Could you check a few things on this model? Use its own coordinates, in mm. Coordinates: 2 decimals unless noted, no trailing zeros. Write each loop counter-clockwise with the first axis right and the second up, starting at its lowest first coordinate (ties: lowest second). Pieces come first, ordered by that corner, then holes. Notation, with made-up numbers: (86, -21) - (125, -21) arc R30 cw to (125, 8) - close; hole circle Ø2 at (20.25, 53). An arc over 180 degrees is marked (long way). Answer as a JSON object with one key per item and string values. Group by question number.
1) Please list where these lines run through material, in increasing order: line 1 along X through (y, z) = (1.85, 0); line 2 along Z through (x, y) = (45, 1.2); line 3 along X through (y, z) = (1.6, 1.5).
2) If we section it at B-B (y = 1.8): Write out the boundary of the cut face in (x, z).
3) Will this pin go through, and if not, where does the flat tip stop? pin 1 Ø6.5 at (x, z) = (45, 0) entering from +Y.
4) If we section it at A-A (z = 0): Write out the boundary of the cut face in (x, y), plus the area to 3 significant figures.
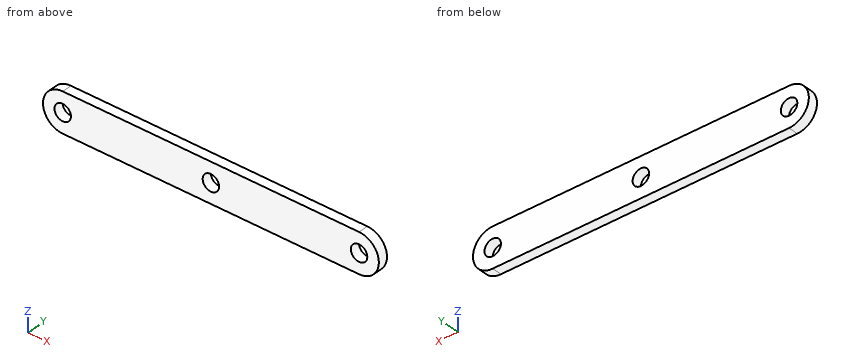
```python
from build123d import *

# Parameters (mm, degrees)
EXTRUDE_1_DEPTH     = 3
CUT_EXTRUDE_1_REACH = 5
SKETCH_2_R          = 2.5


with BuildPart() as part:
    # 草圖1 → 填料-伸長1 (new body)
    with BuildSketch(Plane(origin=(0, 0, 0), x_dir=(1, 0, 0), z_dir=(0, 1, 0))):
        with BuildLine():
            Line((-45, 6), (45, 6))
            ThreePointArc((45, 6), (51, 0), (45, -6))
            Line((45, -6), (-45, -6))
            ThreePointArc((-45, -6), (-51, 0), (-45, 6))
        make_face()
    extrude(amount=EXTRUDE_1_DEPTH)

    # 草圖2 → 除料-伸長1 (cut, up to next)
    with BuildSketch(Plane(origin=(0, 3, 0), x_dir=(1, 0, 0), z_dir=(0, 1, 0)), mode=Mode.PRIVATE) as cut_extrude_1_sk1:
        with Locations((-45, 0)):
            Circle(SKETCH_2_R)
    cut_extrude_1_tool1 = extrude(cut_extrude_1_sk1.sketch, amount=-CUT_EXTRUDE_1_REACH, mode=Mode.PRIVATE) & part.part
    add(cut_extrude_1_tool1.solids().sort_by_distance((-45, 3, 0))[0], mode=Mode.SUBTRACT)
    # 草圖2 → 除料-伸長1 (cut, up to next)
    with BuildSketch(Plane(origin=(0, 3, 0), x_dir=(1, 0, 0), z_dir=(0, 1, 0)), mode=Mode.PRIVATE) as cut_extrude_1_sk2:
        with Locations((45, 0)):
            Circle(SKETCH_2_R)
    cut_extrude_1_tool2 = extrude(cut_extrude_1_sk2.sketch, amount=-CUT_EXTRUDE_1_REACH, mode=Mode.PRIVATE) & part.part
    add(cut_extrude_1_tool2.solids().sort_by_distance((45, 3, 0))[0], mode=Mode.SUBTRACT)
    # 草圖2 → 除料-伸長1 (cut, up to next)
    with BuildSketch(Plane(origin=(0, 3, 0), x_dir=(1, 0, 0), z_dir=(0, 1, 0)), mode=Mode.PRIVATE) as cut_extrude_1_sk3:
        Circle(SKETCH_2_R)
    cut_extrude_1_tool3 = extrude(cut_extrude_1_sk3.sketch, amount=-CUT_EXTRUDE_1_REACH, mode=Mode.PRIVATE) & part.part
    add(cut_extrude_1_tool3.solids().sort_by_distance((0, 3, 0))[0], mode=Mode.SUBTRACT)


solid = part.part
```
Here are the results:
{
 "1": {"line 1": "x = -51 to -47.5, -42.5 to -2.5, 2.5 to 42.5, 47.5 to 51", "line 2": "z = -6 to -2.5, 2.5 to 6", "line 3": "x = -50.81 to -47, -43 to -2, 2 to 43, 47 to 50.81"},
 "2": {"outline": "(-45, -6) - (45, -6) arc R6 ccw to (45, 6) - (-45, 6) arc R6 ccw to start; hole circle Ø5 at (-45, 0); hole circle Ø5 at (0, 0); hole circle Ø5 at (45, 0)"},
 "3": {"pin 1": "stops at y = 3"},
 "4": {"outline": "(-51, 0) - (-47.5, 0) - (-47.5, 3) - (-51, 3) - close; (-42.5, 0) - (-2.5, 0) - (-2.5, 3) - (-42.5, 3) - close; (2.5, 0) - (42.5, 0) - (42.5, 3) - (2.5, 3) - close; (47.5, 0) - (51, 0) - (51, 3) - (47.5, 3) - close", "area": "261 mm²"}
}
